Source: CAD feature listing. Evaluate the final solid. Frame: model axes, mm. A direction names the side the tool comes from. Coordinates: 2 decimals unless noted, no trailing zeros. Order: outer loops, then holes, each group sorted by start corner. A loop starts at its lowest first (then second) coordinate and runs counter-clockwise, first axis right, second up.
```python
from build123d import *

# Parameters (mm, degrees)
F1_DEPTH = 4


with BuildPart() as f1:
    # F0 (on Right) → F1 (new body)
    with BuildSketch(Plane.YZ):
        with BuildLine():
            Line((0, 67.3), (0, 0))
            Line((0, 0), (55.40454, 0))
            ThreePointArc((55.40454, 0), (65.797372, 1.979846), (75.582232, 6.003182))
            Line((75.582232, 6.003182), (75.582232, 14.138489))
            Line((75.582232, 14.138489), (13.826331, 14.138489))
            Line((13.826331, 14.138489), (13.826331, 54.936416))
            Line((13.826331, 54.936416), (65.826331, 54.936416))
            Line((65.826331, 54.936416), (65.826331, 67.3))
            Line((65.826331, 67.3), (0, 67.3))
        make_face()
    extrude(amount=F1_DEPTH)


solid = f1.part
```
1. Section query C-C on z = 38.5. Return loops of the section in (x, y), plus the area to 3 significant figures.
Findings:
outline: (0, 0) - (4, 0) - (4, 13.83) - (0, 13.83) - close
area: 55.3 mm2
2. Pin query (flat end, axial travel): P1, Ø1.2, axis at x = 1.5, z = 63, coming from the +Y side; P2, Ø2, axis at x = 1.5, z = 32.5, coming from the +Y side. Return the tip coordinate at first contact, or that it passes through.
Findings:
P1: stops at y = 65.83
P2: stops at y = 13.83
3. Ray query, line 1 (Z direction, x = 1.75, y = 45); line 2 (Y direction, x = 0.8, z = 32.5); line 3 (Y direction, x = 1.25, z = 57.5). Return the intervals inside material, ascending.
Findings:
line 1: z = 0 to 14.14, 54.94 to 67.3
line 2: y = 0 to 13.83
line 3: y = 0 to 65.83
4. Section query D-D on y = 34. Return loops of the section in (x, z).
Findings:
outline: (0, 0) - (4, 0) - (4, 14.14) - (0, 14.14) - close; (0, 54.94) - (4, 54.94) - (4, 67.3) - (0, 67.3) - close
5. Section query B-B on x = 2.9. Return loops of the section in (y, z).
Findings:
outline: (0, 0) - (55.4, 0) arc R52.5 ccw to (75.58, 6) - (75.58, 14.14) - (13.83, 14.14) - (13.83, 54.94) - (65.83, 54.94) - (65.83, 67.3) - (0, 67.3) - close
6. Section query A-A on y = 56.5. Return loops of the section in (x, z), plus the area to 3 significant figures.
Findings:
outline: (0, 0.11) - (4, 0.11) - (4, 14.14) - (0, 14.14) - close; (0, 54.94) - (4, 54.94) - (4, 67.3) - (0, 67.3) - close
area: 106 mm2
7. Access query for faces 1 (the face through (2, 45, 14.138)), 2 (the face through (4, 12, 34)), 3 (the face through (2, 65.826, 61)). Directions: +Z, -Z, +X, -X, +Y, -Y. A direction counts if a zero-diameter tool reaches every point of the face in a straight line with its end or side. Return the directions, or none.
Findings:
face 1: +X, -X, +Y
face 2: +Z, -Z, +X, +Y, -Y
face 3: +Z, +X, -X, +Y
8. Draft query along Z for faces 4 (the face through (2, 39, 54.936)), 5 (the face through (1.97, 65.66, 1.94)), 6 (the face through (0, 12, 34)). Return one class per face: released by +Z, released by -Z, zero draft, split by the parting line, or undercut.
Findings:
face 4: undercut
face 5: released by -Z
face 6: zero draft
